from build123d import *

# Parameters (mm, degrees)
SKETCH1_W           = 431.8
SKETCH1_H           = 63.5
BOSS_EXTRUDE1_DEPTH = 19.05
CUT_EXTRUDE2_DEPTH  = 220.051991545
CUT_EXTRUDE1_DEPTH  = 19.05
SKETCH5_W           = 241.3
SKETCH5_H           = 19.05
CUT_EXTRUDE3_DEPTH  = 9.525


with BuildPart() as part:
    # Sketch1 → Boss-Extrude1 (new body)
    with BuildSketch(Plane(origin=(0, 0, 0), x_dir=(1, 0, 0), z_dir=(0, 1, 0))):
        Rectangle(SKETCH1_W, SKETCH1_H)
    extrude(amount=BOSS_EXTRUDE1_DEPTH)

    # Sketch3 → Cut-Extrude2 (cut, through all)
    with BuildSketch(Plane(origin=(0, 19.05, 0), x_dir=(1, 0, 0), z_dir=(0, 1, 0))):
        Polygon((-215.9, 31.75), (-190.5, -31.75), (-215.9, -31.75), align=None)
        Polygon((215.9, 0), (138.43, -31.75), (215.9, -31.75), align=None)
    extrude(amount=-CUT_EXTRUDE2_DEPTH, mode=Mode.SUBTRACT)

    # Sketch2 → Cut-Extrude1 (cut)
    with BuildSketch(Plane(origin=(0, 19.05, 0), x_dir=(1, 0, 0), z_dir=(0, 1, 0))):
        with BuildLine():
            Line((158.75, -4.064), (120.65, -4.064))
            ThreePointArc((120.65, -4.064), (116.586, 0), (120.65, 4.064))
            Line((120.65, 4.064), (158.75, 4.064))
            ThreePointArc((158.75, 4.064), (162.814, 0), (158.75, -4.064))
        make_face()
        with BuildLine():
            Line((-184.15, 4.064), (-146.05, 4.064))
            ThreePointArc((-146.05, 4.064), (-141.986, 0), (-146.05, -4.064))
            Line((-146.05, -4.064), (-184.15, -4.064))
            ThreePointArc((-184.15, -4.064), (-188.214, 0), (-184.15, 4.064))
        make_face()
    extrude(amount=-CUT_EXTRUDE1_DEPTH, mode=Mode.SUBTRACT)

    # Sketch5 → Cut-Extrude3 (cut)
    with BuildSketch(Plane(origin=(0, 19.05, 0), x_dir=(1, 0, 0), z_dir=(0, 1, 0))):
        with Locations((-12.7, 0)):
            Rectangle(SKETCH5_W, SKETCH5_H)
    extrude(amount=-CUT_EXTRUDE3_DEPTH, mode=Mode.SUBTRACT)


solid = part.part
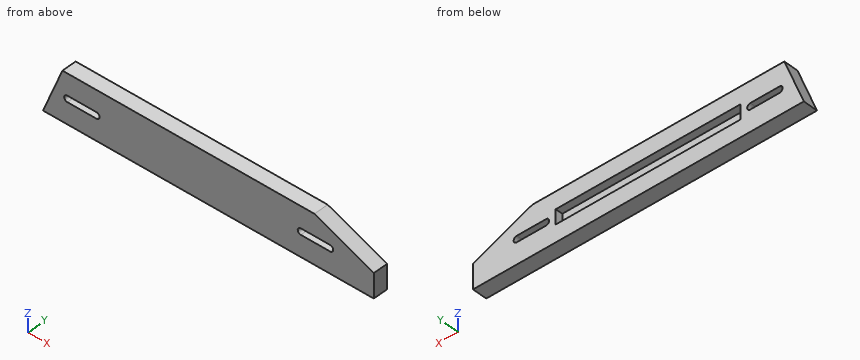
The listing builds one solid part. Answer for the finished solid, in the listing's coordinates (mm). Coordinates: 2 decimals unless noted, no trailing zeros. Order: outer loops, then holes, each group sorted by start corner. A loop starts at its lowest first (then second) coordinate and runs counter-clockwise, first axis right, second up. Notation, with made-up numbers: (78, 46) -> (126, 46) arc R24 cw to (126, 59) -> close; hole circle Ø9 at (86.25, 62.25). An arc over 180 degrees is marked (long way). Answer in a Markdown table with one row per item. Add a question column.
Item 1: Find the intervals of material crossed by L1, parallel to Z at x = 30, y = 10.5 (3 decimals); L2, parallel to Z at x = -153.5, y = 7; L3, parallel to X at y = 14.25, z = -3.5, in increasing order. Write a range as from..to.
Item 2: Find section C-C (z = 13.5). Write down the section's boundary in (x, y), then the cut area to 3 significant figures.
Item 3: Find section D-D (x = 3). Write down the section's boundary in (y, z) (3 decimals).
Item 4: Find section B-B (x = 145.5). Write down the section's boundary in (y, z), then the cut area to 4 significant figures.
Item 5: Each of these flat-tipped pins is pushed along its axis until it touches: P1, Ø4, axis at y = 13, z = 11, coming from the -X side; P2, Ø1.5, axis at y = 2, z = -2.5, coming from the -X side; P3, Ø5, axis at y = 15.5, z = -2.5, coming from the -X side. Where does it stop, or does it pass through?
Item 6: Find section A-A (y = 3.25). Write down the section's boundary in (x, z), then the cut area to 3 significant figures.
Result set:
| question | item | result |
|---|---|---|
| 1 | L1 | z = -31.75..-9.525, 9.525..31.75 |
| 1 | L2 | z = -31.75..-4.06, 4.06..31.75 |
| 1 | L3 | x = -204.6..-186.22, -143.98..-133.35, 107.95..118.58, 160.82..215.9 |
| 2 | outline | (-197.8, 0) -> (182.96, 0) -> (182.96, 19.05) -> (-197.8, 19.05) -> close |
| 2 | area | 7,250 mm² |
| 3 | outline | (0, -31.75) -> (19.05, -31.75) -> (19.05, -9.525) -> (9.525, -9.525) -> (9.525, 9.525) -> (19.05, 9.525) -> (19.05, 31.75) -> (0, 31.75) -> close |
| 4 | outline | (0, -31.75) -> (19.05, -31.75) -> (19.05, -4.06) -> (0, -4.06) -> close; (0, 4.06) -> (19.05, 4.06) -> (19.05, 28.85) -> (0, 28.85) -> close |
| 4 | area | 1,000 mm² |
| 5 | P1 | stops at x = -199.6 |
| 5 | P2 | stops at x = -204.5 |
| 5 | P3 | stops at x = -205.2 |
| 6 | outline | (-215.9, -31.75) -> (215.9, -31.75) -> (215.9, 0) -> (138.43, 31.75) -> (-190.5, 31.75) -> close; hole (-184.15, -4.06) -> (-146.05, -4.06) arc R4.06 ccw to (-146.05, 4.06) -> (-184.15, 4.06) arc R4.06 ccw to start; hole (120.65, -4.06) -> (158.75, -4.06) arc R4.06 ccw to (158.75, 4.06) -> (120.65, 4.06) arc R4.06 ccw to start |
| 6 | area | 24,700 mm² |
